Design review of the part built by this model. Coordinates are the model's own, in mm. A direction names the side the tool comes from. Coordinates: 2 decimals unless noted, no trailing zeros. Loops run counter-clockwise (first coordinate to the right, second up) from the corner with the lowest first, then second, coordinate; pieces in that order, holes last. Notation, with made-up numbers: M -23.75,70.25 L -19.75,70.25 A23 cw -19.75,78.25 Z; hole C 74,64.5 d9. An arc over 180 degrees is marked long. Answer as a JSON object with one key per item and string values. Group by question number.
1. Consider section B-B (x = 55). State the section outline as (y, z) points, then the cut area to 3 significant figures.
2. Consider section D-D (x = -4.5). State the section outline as (y, z) points.
3. Machinability: for faces 1 (the cylindrical face through (330.723, -23.198, 0.49)), 2 (the cylindrical face through (-39.99, -0.88, 40.07)), 3 (the flat face through (189, 25, -40)), which of the approach directions +Z, -Z, +X, -X, +Y, -Y give a long, thin tool a straight path to every point of the face, cutting with its end or side? Answer none if there is none.
4. Insertion check: pin 1 (8 mm diameter, centred on y = 27.5, z = -36, fed in from -X). The pin has a flat end and moves straight along its axis. Give the tip position at first contact, or say it passes through.
5. To check wall thickness, follow probe 1 along Y at (x, z) = (380, 42); probe 2 along Z at (x, y) = (244, 34); probe 3 along Y at (x, z) = (160, -41). State the ranges of each line that lie inside material, in increasing order.
6. Draft analysis for pull direction X (two halves, no side actions). For faces 4 (the flat face through (187, -26, 45)), 5 (the cylindrical face through (49, -25, 0)), 6 (the cylindrical face through (419.99, 0.88, 40.07)), state which applies: +X half, -X half, draft (parallel to the pull), parting line (faces both ways), or undercut.
7. Consider section A-A (y = 0). Count the separate pieces of the cut face and the enclosed holes in it, then the cut area to 3 significant figures.
8. Consider section C-C (z = 39). State the section outline as (x, y) points.
from build123d import *

# Parameters (mm, degrees)
SKETCH2_R           = 30
BOSS_EXTRUDE1_DEPTH = 52.5
BOSS_EXTRUDE2_DEPTH = 10
CUT_EXTRUDE1_DEPTH  = 434.01991871
SKETCH5_R           = 30
BOSS_EXTRUDE3_DEPTH = 52.5
SKETCH7_R           = 6
BOSS_EXTRUDE4_DEPTH = 80
SKETCH8_R           = 30
CUT_EXTRUDE2_DEPTH  = 435.770054167


with BuildPart() as part:
    # Sketch2 → Boss-Extrude1 (new, symmetric)
    with BuildSketch(Plane.XY):
        Circle(SKETCH2_R)
    extrude(amount=BOSS_EXTRUDE1_DEPTH, both=True)

    # Sketch3 → Boss-Extrude2 (add)
    with BuildSketch(Plane.XY.offset(45)):
        with BuildLine():
            Line((0, 40), (380, 40))
            ThreePointArc((380, 40), (420, 0), (380, -40))
            Line((380, -40), (0, -40))
            ThreePointArc((0, -40), (-40, 0), (0, 40))
        make_face()
    boss_extrude2 = extrude(amount=-BOSS_EXTRUDE2_DEPTH)

    # Sketch4 → Cut-Extrude1 (cut, through all)
    with BuildSketch(Plane.XY.offset(45)):
        with BuildLine():
            Line((265, -25), (115, -25))
            ThreePointArc((115, -25), (90, 0), (115, 25))
            Line((115, 25), (265, 25))
            ThreePointArc((265, 25), (290, 0), (265, -25))
        make_face()
    cut_extrude1 = extrude(amount=-CUT_EXTRUDE1_DEPTH, mode=Mode.SUBTRACT)

    # Sketch5 → Boss-Extrude3 (add, symmetric)
    with BuildSketch(Plane.XY):
        with Locations((380, 0)):
            Circle(SKETCH5_R)
    extrude(amount=BOSS_EXTRUDE3_DEPTH, both=True)

    # Mirror1: Boss-Extrude2, Cut-Extrude1 across plane
    add(boss_extrude2.mirror(Plane.XY))
    add(cut_extrude1.mirror(Plane.XY), mode=Mode.SUBTRACT)

    # Sketch7 → Boss-Extrude4 (add)
    with BuildSketch(Plane.XY.offset(45)):
        with Locations((55, 25)):
            Circle(SKETCH7_R)
        with Locations((325, 25)):
            Circle(SKETCH7_R)
        with Locations((325, -25)):
            Circle(SKETCH7_R)
        with Locations((55, -25)):
            Circle(SKETCH7_R)
    extrude(amount=-BOSS_EXTRUDE4_DEPTH)

    # Sketch8 → Cut-Extrude2 (cut, through all)
    with BuildSketch(Plane.XY.offset(52.5)):
        Circle(SKETCH8_R)
        with Locations((380, 0)):
            Circle(SKETCH8_R)
    extrude(amount=-CUT_EXTRUDE2_DEPTH, mode=Mode.SUBTRACT)


solid = part.part
Findings below:
{
 "1": {"outline": "M -40,-45 L 40,-45 L 40,-35 L 31,-35 L 31,35 L 40,35 L 40,45 L -40,45 L -40,35 L -31,35 L -31,-35 L -40,-35 Z; hole M -19,-35 L 19,-35 L 19,35 L -19,35 Z", "area": "3,280 mm^2"},
 "2": {"outline": "M -39.75,-45 L -29.66,-45 L -29.66,-35 L -39.75,-35 Z; M -39.75,35 L -29.66,35 L -29.66,45 L -39.75,45 Z; M 29.66,-45 L 39.75,-45 L 39.75,-35 L 29.66,-35 Z; M 29.66,35 L 39.75,35 L 39.75,45 L 29.66,45 Z"},
 "3": {"face 1": "none", "face 2": "+Z, -Z, -X", "face 3": "+Z, -Z"},
 "4": {"pin 1": "stops at x = -32.37"},
 "5": {"probe 1": "y = -40 to -30, 30 to 40", "probe 2": "z = -45 to -35, 35 to 45", "probe 3": "y = -40 to -25, 25 to 40"},
 "6": {"face 4": "draft", "face 5": "undercut", "face 6": "+X half"},
 "7": {"separate pieces": "8", "enclosed holes": "0", "area": "2,800 mm^2"},
 "8": {"outline": "M 0,-40 L 380,-40 A40 ccw 380,40 L 0,40 A40 ccw Z; hole C 0,0 d60; hole M 115,-25 L 265,-25 A25 ccw 265,25 L 115,25 A25 ccw Z; hole C 380,0 d60"}
}
